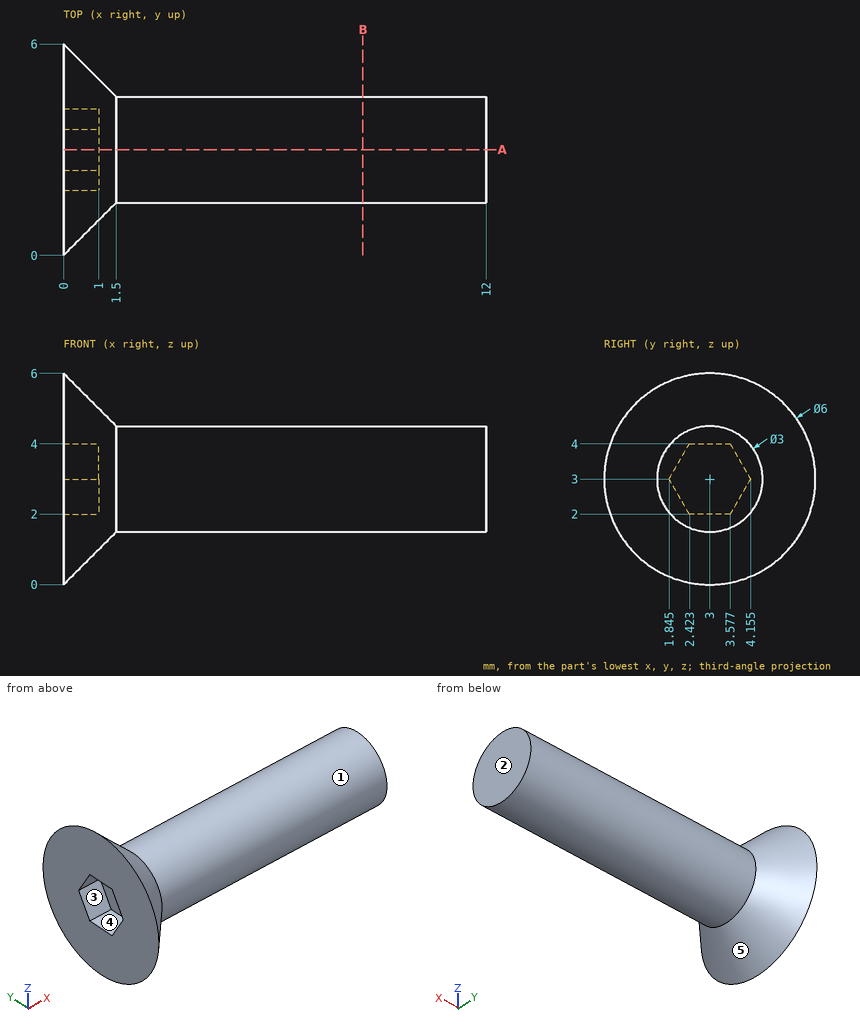
Input: dimensioned drawing with shaded views. Units: mm. Origin: part minimum x, y, z. A direction names the side the tool comes from. Round coordinates to 2 decimals unless told otherwise and drop trailing zeros. Order: outer loops, then holes, each group sorted by start corner. A loop starts at its lowest first (then second) coordinate and runs counter-clockwise, first axis right, second up. Notation, with made-up numbers: (70.5, 52) -> (129.5, 52) arc R8 ccw to (129.5, 56) -> close; hole circle Ø3 at (3, 83.5). An arc over 180 degrees is marked (long way). One line per item, written item: value. Start each with the question number.
Q1. Pin query (flat end, axial travel): pin 1 (1.5 mm diameter, centred on y = 5.5, z = 3.5, fed in from +X); pin 2 (1 mm diameter, centred on x = 2.5, z = 4.5, fed in from -Y); pin 3 (2 mm diameter, centred on x = 2, z = 3.5, fed in from +Y). Return the tip coordinate at first contact, or that it passes through.
Q2. Access query for the marked faces 4 and 5. Directions: +Z, -Z, +X, -X, +Y, -Y. A direction counts if a zero-diameter tool reaches every point of the face in a straight line with its end or side. Return the directions, or none.
Q3. Section query A-A (y = 3). Return the cut outline in (x, z).
Q4. Draft query along Z for the marked faces 1, 2 and 3. Return one class per face: pulls with the +Z half, pulls with the -Z half, needs draft (parallel to the pull), parting line crosses it, or undercut.
Q5. Section query B-B (x = 8.5). Return the cut outline in (y, z).
Q6. Material intervals for probe 1 along Y at (x, z) = (9.5, 3.05); probe 2 along X at (y, z) = (3.65, 3.75); probe 3 along Y at (x, z) = (2, 3.5) (1 decimal), sorted ascending.
Findings below:
1. pin 1: x = 1.2
1. pin 2: y = 1.88
1. pin 3: y = 4.96
2. face 4: -X
2. face 5: +X
3. outline: (0, 0) -> (1.5, 1.5) -> (12, 1.5) -> (12, 4.5) -> (1.5, 4.5) -> (0, 6) -> (0, 4) -> (1, 4) -> (1, 2) -> (0, 2) -> close
4. face 1: parting line crosses it
4. face 2: needs draft
4. face 3: undercut
5. outline: circle Ø3 at (3, 3)
6. probe 1: 1.5 to 4.5
6. probe 2: 1 to 12
6. probe 3: 1.6 to 4.4
